from build123d import *

# Parameters (mm, degrees)
SKETCH1_W           = 150
SKETCH1_H           = 36
BOSS_EXTRUDE1_DEPTH = 70
SKETCH3_W           = 148
SKETCH3_H           = 68
CUT_EXTRUDE1_DEPTH  = 111.180351821
SKETCH4_W           = 35
SKETCH4_H           = 70
BOSS_EXTRUDE3_DEPTH = 1
SKETCH5_W           = 80
SKETCH5_H           = 25
BOSS_EXTRUDE4_DEPTH = 70
SKETCH6_W           = 78
SKETCH6_H           = 68
CUT_EXTRUDE2_DEPTH  = 24


with BuildPart() as part:
    # Sketch1 → Boss-Extrude1 (new body)
    with BuildSketch(Plane.XY):
        with Locations((2.095459837, 17.011641444)):
            Rectangle(SKETCH1_W, SKETCH1_H)
    extrude(amount=BOSS_EXTRUDE1_DEPTH)

    # Sketch3 → Cut-Extrude1 (cut, through all)
    with BuildSketch(Plane(origin=(0, 35.011641444, 0), x_dir=(1, 0, 0), z_dir=(0, 1, 0))):
        with Locations((2.095459837, -35)):
            Rectangle(SKETCH3_W, SKETCH3_H)
    extrude(amount=-CUT_EXTRUDE1_DEPTH, mode=Mode.SUBTRACT)

    # Sketch4 → Boss-Extrude3 (add)
    with BuildSketch(Plane(origin=(0, 35.011641444, 0), x_dir=(1, 0, 0), z_dir=(0, 1, 0))):
        with Locations((59.595459837, -35)):
            Rectangle(SKETCH4_W, SKETCH4_H)
        with Locations((-55.404540163, -35)):
            Rectangle(SKETCH4_W, SKETCH4_H)
    extrude(amount=BOSS_EXTRUDE3_DEPTH)

    # Sketch5 → Boss-Extrude4 (add)
    with BuildSketch(Plane(origin=(0, 0, 0), x_dir=(-1, 0, 0), z_dir=(0, 0, -1))):
        with Locations((-2.095459837, 47.511641444)):
            Rectangle(SKETCH5_W, SKETCH5_H)
    extrude(amount=-BOSS_EXTRUDE4_DEPTH)

    # Sketch6 → Cut-Extrude2 (cut)
    with BuildSketch(Plane.XZ.offset(-35.011641444)):
        with Locations((2.095459837, 35)):
            Rectangle(SKETCH6_W, SKETCH6_H)
    extrude(amount=-CUT_EXTRUDE2_DEPTH, mode=Mode.SUBTRACT)


solid = part.part
CAD build for the part. Positions are in the model's coordinates, mm. A direction names the side the tool comes from. Coordinates: 2 decimals unless noted, no trailing zeros. Write each loop counter-clockwise with the first axis right and the second up, starting at its lowest first coordinate (ties: lowest second). Pieces come first, ordered by that corner, then holes. Notation, with made-up numbers: M -15,-21.5 L 42,-21.5 A15 ccw 42,-13.5 Z; hole C 30,60 d6. An arc over 180 degrees is marked long. Answer as a JSON object with one key per item and string values. Group by question number.
1) Wall check: line 1 (Z direction, x = -8, y = 52); line 2 (X direction, y = 14.5, z = 62); line 3 (X direction, y = 42.5, z = 9). Give the ranges that are in metal, low to high. Write a range as from..to.
2) Mould opens along X. For faces 4 (the face through (77.095, 17, 35)), 5 (the face through (59, 36.012, 35)), 6 (the face through (76.095, 17, 35)) say: +X half, -X half, draft (parallel to the pull), parting line (faces both ways), or undercut.
3) Saw through at C-C (x = 56). Write the cut outline in (y, z), plus the area to 3 significant figures.
4) Saw through at D-D (y = 54). Write the cut outline in (x, z).
5) Saw through at B-B (z = 29). Write the cut outline in (x, y), plus the area to 3 significant figures.
6) Saw through at A-A (y = 15.5). Write the cut outline in (x, z), plus the area to 3 significant figures.
7) Tool access for faces 1 (the face through (-36.905, 47, 35)), 2 (the face through (-56, 36.012, 35)), 3 (the face through (42.095, 48, 35)): list every direction of +Z, -Z, +X, -X, +Y, -Y with a clear straight run to the whole face (end or side of a thin tool).
8) Pin check, flat tips, straight feed: pin 1 Ø3 at (y, z) = (43.5, 33.5) entering from +X; pin 2 Ø10.5 at (x, z) = (52, 22) entering from -Y; pin 3 Ø7 at (y, z) = (44.5, 26.5) entering from -X. Stop position of each tip, or through.
Values follow:
{
 "1": {"line 1": "z = 0..1, 69..70", "line 2": "x = -72.9..-71.9, 76.1..77.1", "line 3": "x = -37.9..-36.9, 41.1..42.1"},
 "2": {"face 4": "+X half", "face 5": "draft", "face 6": "undercut"},
 "3": {"outline": "M -0.99,0 L 36.01,0 L 36.01,70 L -0.99,70 L -0.99,69 L 35.01,69 L 35.01,1 L -0.99,1 Z", "area": "142 mm2"},
 "4": {"outline": "M -37.9,0 L 42.1,0 L 42.1,70 L -37.9,70 Z; hole M -36.9,1 L 41.1,1 L 41.1,69 L -36.9,69 Z"},
 "5": {"outline": "M -72.9,-0.99 L -71.9,-0.99 L -71.9,35.01 L -36.9,35.01 L -36.9,59.01 L 41.1,59.01 L 41.1,35.01 L 76.1,35.01 L 76.1,-0.99 L 77.1,-0.99 L 77.1,36.01 L 42.1,36.01 L 42.1,60.01 L -37.9,60.01 L -37.9,36.01 L -72.9,36.01 Z", "area": "270 mm2"},
 "6": {"outline": "M -72.9,0 L 77.1,0 L 77.1,70 L -72.9,70 Z; hole M -71.9,1 L 76.1,1 L 76.1,69 L -71.9,69 Z", "area": "436 mm2"},
 "7": {"face 1": "-Y", "face 2": "+Z, -Z, -X, +Y", "face 3": "+Z, -Z, +X, +Y"},
 "8": {"pin 1": "stops at x = 42.1", "pin 2": "stops at y = 35.01", "pin 3": "stops at x = -37.9"}
}
